Part model, mm, in its own coordinate system. A direction names the side the tool comes from. Give positions to 0.01 mm unless a question says otherwise; leave off trailing zeros. Loops run counter-clockwise (first coordinate to the right, second up) from the corner with the lowest first, then second, coordinate; pieces in that order, holes last. Notation, with made-up numbers: M 41.25,6.25 L 94.25,6.25 A31 ccw 94.25,37.25 Z; hole C 37.5,67.25 d9. An arc over 180 degrees is marked long. Answer in a Markdown table with one row per item.
from build123d import *

# Parameters (mm, degrees)
EXTRUDE_1_DEPTH              = 10
EXTRUDE_3_DEPTH              = 20
EXTRUDE_4_DEPTH              = 10
SKETCH_4_R                   = 11
EXTRUDE_5_DEPTH              = 2
SKETCH_5_R                   = 2.5
EXTRUDE_6_DEPTH              = 18
SKETCH_6_W                   = 19
SKETCH_6_H                   = 10
EXTRUDE_7_DEPTH              = 6.7
CUT_EXTRUDE_1_DEPTH          = 10
HOLE_WIZARD_M3_1_D           = 2.5
HOLE_WIZARD_M3_1_DEPTH       = 14
HOLE_WIZARD_M3_1_CBORE_D     = 5.5
HOLE_WIZARD_M3_1_CBORE_DEPTH = 4.5
HOLE_WIZARD_M3_1_TIP         = 0.751075774


with BuildPart() as part:
    # 草图1 → 凸台-拉伸1 (new body)
    with BuildSketch(Plane(origin=(0, 0, 0), x_dir=(1, 0, 0), z_dir=(0, 1, 0))):
        Polygon((-21, 18), (-18, 21), (18, 21), (21, 18), (21, -18), (18, -21), (-18, -21), (-21, -18), align=None)
    extrude(amount=EXTRUDE_1_DEPTH)

    # 草图2 → 凸台-拉伸3 (add)
    with BuildSketch(Plane(origin=(0, 10, 0), x_dir=(1, 0, 0), z_dir=(0, 1, 0))):
        Polygon((21.5, 18.207106781), (18.207106781, 21.5), (-18.207106781, 21.5), (-21.5, 18.207106781), (-21.5, -18.207106781), (-18.207106781, -21.5), (18.207106781, -21.5), (21.5, -18.207106781), align=None)
    extrude(amount=EXTRUDE_3_DEPTH)

    # 草图3 → 凸台-拉伸4 (add)
    with BuildSketch(Plane(origin=(0, 30, 0), x_dir=(1, 0, 0), z_dir=(0, 1, 0))):
        Polygon((21, -18), (21, 18), (18, 21), (-18, 21), (-21, 18), (-21, -18), (-18, -21), (18, -21), align=None)
    extrude(amount=EXTRUDE_4_DEPTH)

    # 草图4 → 凸台-拉伸5 (add)
    with BuildSketch(Plane(origin=(0, 40, 0), x_dir=(1, 0, 0), z_dir=(0, 1, 0))):
        Circle(SKETCH_4_R)
    extrude(amount=EXTRUDE_5_DEPTH)

    # 草图5 → 凸台-拉伸6 (add)
    with BuildSketch(Plane(origin=(0, 42, 0), x_dir=(1, 0, 0), z_dir=(0, 1, 0))):
        Circle(SKETCH_5_R)
    extrude(amount=EXTRUDE_6_DEPTH)

    # 草图6 → 凸台-拉伸7 (add)
    with BuildSketch(Plane.XY.offset(21)):
        with Locations((0, 5)):
            Rectangle(SKETCH_6_W, SKETCH_6_H)
    extrude(amount=EXTRUDE_7_DEPTH)

    # 草图7 → 切除-拉伸1 (cut)
    with BuildSketch(Plane(origin=(0, 60, 0), x_dir=(1, 0, 0), z_dir=(0, 1, 0))):
        with BuildLine():
            Line((-1.5, -2), (1.5, -2))
            ThreePointArc((1.5, -2), (0, -2.5), (-1.5, -2))
        make_face()
    extrude(amount=-CUT_EXTRUDE_1_DEPTH, mode=Mode.SUBTRACT)

    # M3 六角头机械螺钉的柱形沉头孔1
    with Locations(Plane(origin=(0, 40, 0), x_dir=(1, 0, 0), z_dir=(0, 1, 0))):
        with Locations((-15.5, 15.5), (15.5, 15.5), (-15.5, -15.5), (15.5, -15.5)):
            CounterBoreHole(HOLE_WIZARD_M3_1_D / 2, HOLE_WIZARD_M3_1_CBORE_D / 2, HOLE_WIZARD_M3_1_CBORE_DEPTH, depth=HOLE_WIZARD_M3_1_DEPTH)
            with Locations((0, 0, -(HOLE_WIZARD_M3_1_DEPTH + HOLE_WIZARD_M3_1_TIP / 2))):  # 118° drill point
                Cone(0, HOLE_WIZARD_M3_1_D / 2, HOLE_WIZARD_M3_1_TIP, mode=Mode.SUBTRACT)


solid = part.part
(1) Drill centre lines: line 1 along X through (y, z) = (28, 15.5); line 2 along Z through (x, y) = (-15.5, 31.75); line 3 along X through (y, z) = (38, -15.5). Where is each one in solid material? Low to high.
Recorded:
| item | result |
|---|---|
| line 1 | x = -21.5 to -16.75, -14.25 to 14.25, 16.75 to 21.5 |
| line 2 | z = -21 to -16.75, -14.25 to 14.25, 16.75 to 21 |
| line 3 | x = -21 to -18.25, -12.75 to 12.75, 18.25 to 21 |
(2) Which spindle directions (+Z, -Z, +X, -X, +Y, -Y) get a long thin tool onto all of the face, cutting with end or side? Do faces 4 (the face through (-20, 5, -19)), 5 (the face through (16, 35.5, 17)), 6 (the face through (0, 35, -21)), 7 (the face through (19, 35, 20)). Say none if no direction does.
Recorded:
| item | result |
|---|---|
| face 4 | -Z, -X, -Y |
| face 5 | +Y |
| face 6 | -Z, +X, -X, +Y |
| face 7 | +Z, +X, +Y |
(3) Saw through at A-A (x = 12). Write the cut outline in (y, z).
Recorded:
| item | result |
|---|---|
| outline | M 0,-21 L 10,-21 L 10,-21.5 L 30,-21.5 L 30,-21 L 40,-21 L 40,21 L 30,21 L 30,21.5 L 10,21.5 L 10,21 L 0,21 Z |
(4) Saw through at D-D (x = -19). Write the cut outline in (y, z), plus the area to 3 significant figures.
Recorded:
| item | result |
|---|---|
| outline | M 0,-20 L 10,-20 L 10,-20.71 L 30,-20.71 L 30,-20 L 40,-20 L 40,20 L 30,20 L 30,20.71 L 10,20.71 L 10,20 L 0,20 Z |
| area | 1,630 mm^2 |
(5) Pin check, flat tips, straight feed: pin 1 Ø1.5 at (x, z) = (-15.5, 15.5) entering from -Y; pin 2 Ø4 at (x, y) = (13.5, 5) entering from +Z; pin 3 Ø3 at (x, z) = (12.5, 13) entering from +Y; pin 4 Ø8 at (y, z) = (42, 12) entering from -X. Stop position of each tip, or through.
Recorded:
| item | result |
|---|---|
| pin 1 | stops at y = 0 |
| pin 2 | stops at z = 21 |
| pin 3 | stops at y = 40 |
| pin 4 | stops at x = -21 |
(6) Saw through at B-B (z = 0). Write the cut outline in (x, y).
Recorded:
| item | result |
|---|---|
| outline | M -21.5,10 L -21,10 L -21,0 L 21,0 L 21,10 L 21.5,10 L 21.5,30 L 21,30 L 21,40 L 11,40 L 11,42 L 2.5,42 L 2.5,60 L -2.5,60 L -2.5,42 L -11,42 L -11,40 L -21,40 L -21,30 L -21.5,30 Z |
(7) Pull direction Z, two halves, no side cores. Call faces 1 (the face through (19.877, 19.86, -19.831)), 2 (the face through (-15.55, 25.38, -15.29)), 3 (the face through (-21, 35, 0)): +Z half, -Z half, draft (parallel to the pull), parting line (faces both ways), or undercut.
Recorded:
| item | result |
|---|---|
| face 1 | -Z half |
| face 2 | undercut |
| face 3 | draft |
(8) Saw through at C-C (x = 0). Write the cut outline in (y, z).
Recorded:
| item | result |
|---|---|
| outline | M 0,-21 L 10,-21 L 10,-21.5 L 30,-21.5 L 30,-21 L 40,-21 L 40,-11 L 42,-11 L 42,-2.5 L 60,-2.5 L 60,2 L 50,2 L 50,2.5 L 42,2.5 L 42,11 L 40,11 L 40,21 L 30,21 L 30,21.5 L 10,21.5 L 10,27.7 L 0,27.7 Z |
